from build123d import *

# Parameters (mm, degrees)
SKETCH1_R           = 10
BOSS_EXTRUDE1_DEPTH = 10
SKETCH1_4_R         = 10
SKETCH1_4_R_2       = 8
BOSS_EXTRUDE2_DEPTH = 15
SKETCH1_5_R         = 10
BOSS_EXTRUDE3_DEPTH = 40
FILLET1_R           = 5
FILLET2_R           = 2


with BuildPart() as part:
    # Sketch1 → Boss-Extrude1 (new body)
    with BuildSketch(Plane(origin=(0, 0, 0), x_dir=(1, 0, 0), z_dir=(0, 1, 0))):
        with BuildLine():
            Line((60, 20), (20, 20))
            Line((20, 20), (20, -20))
            Line((20, -20), (60, -20))
            ThreePointArc((60, -20), (80, 0), (60, 20))
        make_face()
        with Locations(Location((60, 0, 0), (0, 0, 270))):
            Circle(SKETCH1_R, mode=Mode.SUBTRACT)
    extrude(amount=BOSS_EXTRUDE1_DEPTH)

    # Sketch1_4 → Boss-Extrude2 (add)
    with BuildSketch(Plane(origin=(0, 0, 0), x_dir=(1, 0, 0), z_dir=(0, 1, 0))):
        with Locations(Location((60, 0, 0), (0, 0, 270))):
            Circle(SKETCH1_4_R)
        with Locations(Location((60, 0, 0), (0, 0, 270))):
            Circle(SKETCH1_4_R_2, mode=Mode.SUBTRACT)
    extrude(amount=BOSS_EXTRUDE2_DEPTH)

    # Sketch1_5 → Boss-Extrude3 (add)
    with BuildSketch(Plane(origin=(0, 0, 0), x_dir=(1, 0, 0), z_dir=(0, 1, 0))):
        with BuildLine():
            Line((20, 20), (0, 20))
            ThreePointArc((0, 20), (-20, 0), (0, -20))
            Line((0, -20), (20, -20))
            Line((20, -20), (20, 20))
        make_face()
        with Locations(Location((0, 0, 0), (0, 0, 270))):
            Circle(SKETCH1_5_R, mode=Mode.SUBTRACT)
    extrude(amount=BOSS_EXTRUDE3_DEPTH)

    # Fillet1
    fillet1_edges = [part.edges().sort_by_distance(p)[0] for p in [
        (20, 10, 0),
    ]]
    fillet(fillet1_edges, radius=FILLET1_R)

    # Fillet2
    fillet2_edges = [part.edges().sort_by_distance(p)[0] for p in [
        (60, 10, -10),
    ]]
    fillet(fillet2_edges, radius=FILLET2_R)


solid = part.part
Model file for the job. Use its own axes, mm. A direction names the side the tool comes from. Coordinates: 2 decimals unless noted, no trailing zeros. Write each loop counter-clockwise with the first axis right and the second up, starting at its lowest first coordinate (ties: lowest second). Pieces come first, ordered by that corner, then holes. Notation, with made-up numbers: (70.25, 43.25) -> (87.25, 43.25) arc R12 cw to (87.25, 66.25) -> close; hole circle Ø6 at (49.5, 75). An arc over 180 degrees is marked (long way). One line per item, written item: value. Start each with the question number.
1) Slice it at C-C on y = 37.5. Write the cut outline in (x, z).
2) Which spindle directions (+Z, -Z, +X, -X, +Y, -Y) get a long thin tool onto all of the face, cutting with end or side? Do faces 1 (the face through (22, 11, 0)), 2 (the face through (-9.76, 19.72, -2.17)), 3 (the face through (46, 10, 0)), 4 (the face through (17, 15, -20)), 5 (the face through (20, 27, 0)). Say none if no direction does.
3) Slice it at A-A on z = 0. Write the cut outline in (x, y), then the cut area to 3 significant figures.
4) Probe probe 1 along X at (y, z) = (6, 0); probe 2 along X at (y, z) = (10.75, 0); probe 3 along Y at (x, z) = (62, 17.5). List the from-to ranges inside material, lowest first.
5) Pull direction Z, two halves, no side cores. Call faces 6 (the face through (80, 5, 0)), 7 (the face through (67.932, 7.395, -1.041)), 8 (the face through (16, 15, 20)), 9 (the face through (68.2, 15, 0)): +Z half, -Z half, draft (parallel to the pull), parting line (faces both ways), or undercut.
6) Slice it at D-D on y = 6. Write the cut outline in (x, z), then the cut area to 3 significant figures.
7) Slice it at B-B on y = 13. Write the cut outline in (x, z), then the cut area to 3 significant figures.
8) Flat gauge pins, fed straight in: pin 1 Ø5 at (y, z) = (35, -8.5) entering from +X; pin 2 Ø2 at (y, z) = (34.5, -10.5) entering from -X; pin 3 Ø6 at (y, z) = (19, -12) entering from -X. Where does each tip first touch, or does it go through?
Answers follow:
1. outline: (0, -20) -> (20, -20) -> (20, 20) -> (0, 20) arc R20 ccw to start; hole circle Ø20 at (0, 0)
2. face 1: +Z, -Z, +Y
2. face 2: +Y, -Y
2. face 3: +Y
2. face 4: -Z, +X, -X, +Y, -Y
2. face 5: +Z, -Z, +X, +Y
3. outline: (-20, 0) -> (-10, 0) -> (-10, 40) -> (-20, 40) -> close; (10, 0) -> (52, 0) -> (52, 15) -> (50, 15) -> (50, 12) arc R2 cw to (48, 10) -> (25, 10) arc R5 cw to (20, 15) -> (20, 40) -> (10, 40) -> close; (68, 0) -> (80, 0) -> (80, 10) -> (72, 10) arc R2 cw to (70, 12) -> (70, 15) -> (68, 15) -> close
3. area: 1,270 mm2
4. probe 1: -20 to -10, 10 to 52, 68 to 80
4. probe 2: -20 to -10, 10 to 22.37, 49.56 to 52, 68 to 70.44
4. probe 3: 0 to 10
5. face 6: parting line
5. face 7: undercut
5. face 8: +Z half
5. face 9: draft
6. outline: (0, -20) -> (60, -20) arc R20 ccw to (60, 20) -> (0, 20) arc R20 ccw to start; hole circle Ø20 at (0, 0); hole circle Ø16 at (60, 0)
6. area: 3,140 mm2
7. outline: (0, -20) -> (20.42, -20) -> (20.42, 20) -> (0, 20) arc R20 ccw to start; circle Ø20 at (60, 0); hole circle Ø20 at (0, 0); hole circle Ø16 at (60, 0)
7. area: 1,240 mm2
8. pin 1: x = 20
8. pin 2: x = -17.6
8. pin 3: x = -17.86
